Here's how the part is built. I have some questions about the finished solid (model axes, mm). A direction names the side the tool comes from. Round coordinates to 2 decimals unless told otherwise and drop trailing zeros. Write each loop counter-clockwise with the first axis right and the second up, starting at its lowest first coordinate (ties: lowest second). Pieces come first, ordered by that corner, then holes. Notation, with made-up numbers: (66.5, -11.75) - (85.5, -11.75) arc R13 ccw to (85.5, 4.25) - close; hole circle Ø5 at (-15, -23.5). An arc over 180 degrees is marked (long way). Use one line per item in the form item = value. Start each with the question number.
1. Which directions (+Z, -Z, +X, -X, +Y, -Y) give clear straight access to the entire face, cutting with the end or side of a thin tool? Please do faces 1 (the cylindrical face through (12.878, -24.636, 0.724)), 2 (the flat face through (4, -13, 20.32)), 3 (the flat face through (16.1, -12.6, 9.525)).
2. Will these pins go through, and if not, where does the flat tip stop? pin 1 (12.5 mm diameter, centred on x = 12, z = -16, fed in from -Y); pin 2 (2 mm diameter, centred on y = -12.64, z = 16.56, fed in from -X); pin 3 (6 mm diameter, centred on x = 13, y = 0.5, fed in from +Z).
3. If I drill on line 1 along Z through (x, y) = (19.25, -4.5) (3 decimals); line 2 along Y through (x, z) = (12.7, 3.25) (3 decimals); line 3 along Z through (x, y) = (17, -10.5) (3 decimals), over which ranges is the centre line in solid material (lowest first)?
4. I want a section at D-D, the plane y = -12. List the corners of the cut face in (x, z) for me (3 decimals), plus the area to 3 significant figures.
5. I want a section at C-C, the plane y = -1. List the corners of the cut face in (x, z) for me (3 decimals), plus the area to 3 significant figures.
6. I want a section at B-B, the plane x = 12.7. State how many separate pieces and enclosed holes the cut face has, plus the area to 3 significant figures.
7. We'd pull the mould along Z, two halves only. Please class faces 4 (the cylindrical face through (12.878, -24.676, 19.556)), 5 (the flat face through (13, 9.525, -12)), 6 (the flat face through (13, 0, -13)): +Z half, -Z half, draft (parallel to the pull), parting line (faces both ways), or undercut.
```python
from build123d import *

# Parameters (mm, degrees)
BOSS_EXTRUDE1_DEPTH            = 25.4
F_1_4_0_2500_DOWEL_HOLE1_D     = 6.35
F_1_4_0_2500_DOWEL_HOLE1_DEPTH = 20.32
F_10_CLEARANCE_HOLE1_D         = 5.1054
SKETCH8_R                      = 7.9375
CUT_EXTRUDE1_DEPTH             = 10.795
M3X0_5_TAPPED_HOLE1_D          = 2.5
FILLET1_R                      = 2.54


with BuildPart() as part:
    # Sketch1 → Boss-Extrude1 (new body)
    with BuildSketch(Plane(origin=(0, 0, 0), x_dir=(0, 0, -1), z_dir=(1, 0, 0))):
        with BuildLine():
            Line((0, 0), (0, -25.4))
            Line((0, -25.4), (-20.32, -25.4))
            Line((-20.32, -25.4), (-20.32, -3.175))
            ThreePointArc((-20.32, -3.175), (-16.600256121, 5.805256121), (-7.62, 9.525))
            Line((-7.62, 9.525), (34.925, 9.525))
            Line((34.925, 9.525), (34.925, -25.4))
            Line((34.925, -25.4), (25.4, -25.4))
            Line((25.4, -25.4), (25.4, 0))
            Line((25.4, 0), (0, 0))
        make_face()
    extrude(amount=BOSS_EXTRUDE1_DEPTH)

    # 1/4 (0.2500) Dowel Hole1
    with Locations(Plane(origin=(0, 0, 0), x_dir=(-1, 0, 0), z_dir=(0, 0, -1))):
        with Locations((-12.7, -12.7)):
            Hole(F_1_4_0_2500_DOWEL_HOLE1_D / 2, depth=F_1_4_0_2500_DOWEL_HOLE1_DEPTH)

    # #10 Clearance Hole1 (through all)
    with Locations(Plane(origin=(0, 0, -34.925), x_dir=(-1, 0, 0), z_dir=(0, 0, -1))):
        with Locations((-12.7, -12.7)):
            Hole(F_10_CLEARANCE_HOLE1_D / 2)

    # Sketch8 → Cut-Extrude1 (cut)
    with BuildSketch(Plane.XY.offset(20.32)):
        with Locations((12.7, -12.7)):
            Circle(SKETCH8_R)
    extrude(amount=-CUT_EXTRUDE1_DEPTH, mode=Mode.SUBTRACT)

    # M3x0.5 Tapped Hole1 (through all)
    with Locations(Plane(origin=(25.4, 0, 0), x_dir=(0, 0, -1), z_dir=(1, 0, 0))):
        with Locations((-16.5608, -12.6375), (-16.5608, -20.6375)):
            Hole(M3X0_5_TAPPED_HOLE1_D / 2)

    # Fillet1
    fillet1_edges = [part.edges().sort_by_distance(p)[0] for p in [
        (12.7, -25.4, 0),
        (12.7, -25.4, 20.32),
        (12.7, 9.525, -34.925),
        (12.7, -25.4, -34.925),
        (12.7, -25.4, -25.4),
    ]]
    fillet(fillet1_edges, radius=FILLET1_R)


solid = part.part
```
Model answer:
q1.face_1 = +X, -X, -Y
q1.face_2 = +Z, +X, -X, +Y, -Y
q1.face_3 = +Z
q2.pin_1 = 0
q2.pin_2 = through
q2.pin_3 = 20.3
q3.line_1 = -34.925 to -25.4, 0 to 20.32
q3.line_2 = -25.4 to -15.875, -9.525 to 9.525
q3.line_3 = -34.925 to -25.4, 0 to 9.525
q4.outline = (0, -34.925) - (10.245, -34.925) - (10.245, -25.4) - (0, -25.4) - close; (0, 0) - (9.603, 0) - (9.603, 9.525) - (4.793, 9.525) - (4.793, 15.486) - (0, 15.486) - close; (0, 17.636) - (4.793, 17.636) - (4.793, 20.32) - (0, 20.32) - close; (15.155, -34.925) - (25.4, -34.925) - (25.4, -25.4) - (15.155, -25.4) - close; (15.797, 0) - (25.4, 0) - (25.4, 15.486) - (20.607, 15.486) - (20.607, 9.525) - (15.797, 9.525) - close; (20.607, 17.636) - (25.4, 17.636) - (25.4, 20.32) - (20.607, 20.32) - close
q4.area = 461 mm2
q5.outline = (0, -34.925) - (25.4, -34.925) - (25.4, -25.4) - (0, -25.4) - close; (0, 0) - (25.4, 0) - (25.4, 20.132) - (0, 20.132) - close
q5.area = 753 mm2
q6.separate_pieces = 3
q6.enclosed_holes = 0
q6.area = 960 mm2
q7.face_4 = +Z half
q7.face_5 = draft
q7.face_6 = undercut
